Read the model definition and answer for the solid it produces. Units are mm, in the model's axes. Face numbers are marked on the shaded views. A direction names the side the tool comes from. Give positions to 0.01 mm unless a question says otherwise; leave off trailing zeros. Loops run counter-clockwise (first coordinate to the right, second up) from the corner with the lowest first, then second, coordinate; pieces in that order, holes last.
(1) Find section B-B, the plane x = 0. Write down the section's boundary in (y, z), then the cut area to 3 significant figures.
(2) Straight lines are drawn through the part: probe 1 along Y at (x, z) = (-12, -49.5); probe 2 along X at (y, z) = (-18, -48); probe 3 along X at (y, z) = (-12, -13.5). For each, find the intervals that lie inside material, in ascending order.
(3) Find section C-C, the plane x = -8.75. Write down the section's boundary in (y, z).
(4) Find section D-D, the plane y = -3.5. Write down the section's boundary in (x, z), then the cut area to 3 significant figures.
(5) Which of the six approach directions +Z, -Z, +X, -X, +Y, -Y give full straight-line access (tool end or side, diameter ignored) to the marked faces 1, 2, 3, 4 and 5?
(6) Determine the mould class of the marked faces 6, 7 and 8 for opening direction Z: pulls with the +Z half, pulls with the -Z half, needs draft (parallel to the pull), parting line crosses it, or undercut.
(7) Each of these flat-tipped pins is pushed along its axis until it touches: P1, Ø14.5, axis at x = 4, z = -47.5, coming from the +Y side; P2, Ø11, axis at x = -1.5, y = 14.5, coming from the +Z side; P3, Ø3, axis at x = -2.5, z = -17.5, coming from the -Y side; P4, Ø1, axis at x = -11.5, y = -13, coming from the +Z side. Where does it stop, or does it pass through?
(8) Find section A-A, the plane z = -35.5. Write down the section's boundary in (x, y).
```python
from build123d import *

# Parameters (mm, degrees)
SKETCH3_R           = 10
BOSS_EXTRUDE2_DEPTH = 12
BOSS_EXTRUDE3_DEPTH = 5
SKETCH5_R           = 15
BOSS_EXTRUDE4_DEPTH = 4
SKETCH6_W           = 30
SKETCH6_H           = 45
BOSS_EXTRUDE6_DEPTH = 10
BOSS_EXTRUDE7_START = 12.5
SKETCH7_R           = 8
BOSS_EXTRUDE7_DEPTH = 10
BOSS_EXTRUDE8_START = -22.5
SKETCH7_2_R         = 8
BOSS_EXTRUDE8_DEPTH = 10
CUT_EXTRUDE1_REACH  = 80.861


with BuildPart() as part:
    # Sketch3 → Boss-Extrude2 (new, symmetric)
    with BuildSketch(Plane(origin=(0, 0, 0), x_dir=(0, 0, -1), z_dir=(1, 0, 0))):
        Circle(SKETCH3_R)
    extrude(amount=BOSS_EXTRUDE2_DEPTH, both=True)

    # Sketch4 → Boss-Extrude3 (add, symmetric)
    with BuildSketch(Plane(origin=(0, 0, 0), x_dir=(0, 0, -1), z_dir=(1, 0, 0))):
        with BuildLine():
            Line((0, 14), (16, 14))
            Line((16, 14), (16, -14))
            Line((16, -14), (0, -14))
            ThreePointArc((0, -14), (-14, 0), (0, 14))
        make_face()
    extrude(amount=BOSS_EXTRUDE3_DEPTH, both=True)

    # Sketch5 → Boss-Extrude4 (add)
    with BuildSketch(Plane(origin=(0, 0, -16), x_dir=(-1, 0, 0), z_dir=(0, 0, -1))):
        Circle(SKETCH5_R)
    extrude(amount=BOSS_EXTRUDE4_DEPTH)

    # Sketch6 → Boss-Extrude6 (add)
    with BuildSketch(Plane(origin=(0, 0, -20), x_dir=(-1, 0, 0), z_dir=(0, 0, -1))):
        Rectangle(SKETCH6_W, SKETCH6_H)
    extrude(amount=BOSS_EXTRUDE6_DEPTH)

    # Sketch7 → Boss-Extrude7 (add)
    with BuildSketch(Plane(origin=(0, 0, 0), x_dir=(1, 0, 0), z_dir=(0, 1, 0)).offset(BOSS_EXTRUDE7_START)):
        with BuildLine():
            Line((-15, 30), (-15, 48))
            ThreePointArc((-15, 48), (0, 63), (15, 48))
            Line((15, 48), (15, 30))
            Line((15, 30), (-15, 30))
        make_face()
        with Locations(Location((0, 48, 0), (0, 0, 270))):
            Circle(SKETCH7_R, mode=Mode.SUBTRACT)
    extrude(amount=BOSS_EXTRUDE7_DEPTH)

    # Sketch7<2> → Boss-Extrude8 (add)
    with BuildSketch(Plane(origin=(0, 0, 0), x_dir=(1, 0, 0), z_dir=(0, 1, 0)).offset(BOSS_EXTRUDE8_START)):
        with BuildLine():
            Line((-15, 30), (-15, 48))
            ThreePointArc((-15, 48), (0, 63), (15, 48))
            Line((15, 48), (15, 30))
            Line((15, 30), (-15, 30))
        make_face()
        with Locations(Location((0, 48, 0), (0, 0, 270))):
            Circle(SKETCH7_2_R, mode=Mode.SUBTRACT)
    extrude(amount=BOSS_EXTRUDE8_DEPTH)

    # Cut-Extrude1: up to this face of the body (flat: up to its plane)
    cut_extrude1_end = Plane(part.part.faces().sort_by_distance((0, -22.5, -38.416854183))[0])
    # Sketch8 → Cut-Extrude1 (cut, up to the picked face)
    with BuildSketch(Plane(origin=(0, 22.5, 0), x_dir=(1, 0, 0), z_dir=(0, 1, 0)), mode=Mode.PRIVATE) as cut_extrude1_sk1:
        with BuildLine():
            Line((-9.909192751, 59.260901342), (-5.2849028, 54.005814049))
            ThreePointArc((-5.2849028, 54.005814049), (0, 56), (5.2849028, 54.005814049))
            Line((5.2849028, 54.005814049), (9.909192751, 59.260901342))
            ThreePointArc((9.909192751, 59.260901342), (0, 63), (-9.909192751, 59.260901342))
        make_face()
    cut_extrude1_tool1 = split(extrude(cut_extrude1_sk1.sketch, amount=-CUT_EXTRUDE1_REACH, mode=Mode.PRIVATE), bisect_by=cut_extrude1_end, keep=Keep.BOTH, mode=Mode.PRIVATE)
    add(cut_extrude1_tool1.solids().sort_by(Axis((0, 22.5, -58.852599), (0, -1, 0)))[0], mode=Mode.SUBTRACT)


solid = part.part
```
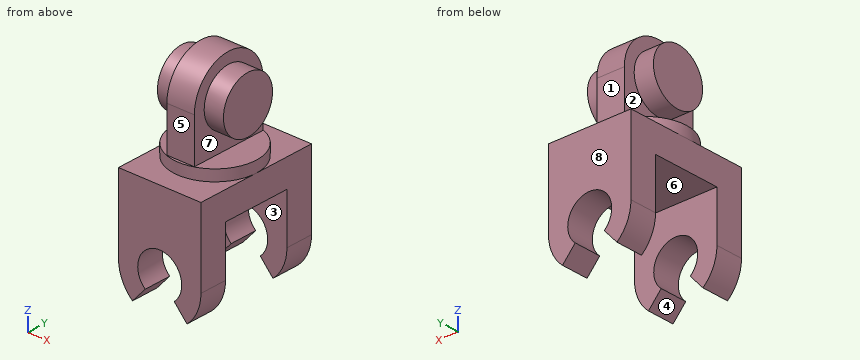
Entries:
1. outline: (-22.5, -40) - (-12.5, -40) - (-12.5, -30) - (12.5, -30) - (12.5, -40) - (22.5, -40) - (22.5, -20) - (15, -20) - (15, -16) - (14, -16) - (14, 0) arc R14 ccw to (-14, 0) - (-14, -16) - (-15, -16) - (-15, -20) - (-22.5, -20) - close
1. area: 1,530 mm2
2. probe 1: y = -22.5 to -12.5, 12.5 to 22.5
2. probe 2: x = -15 to -8, 8 to 15
2. probe 3: x = -5 to 5
3. outline: (-22.5, -57.94) - (-12.5, -57.94) - (-12.5, -30) - (12.5, -30) - (12.5, -57.94) - (22.5, -57.94) - (22.5, -20) - (12.18, -20) - (12.18, -16) - (-12.18, -16) - (-12.18, -20) - (-22.5, -20) - close; circle Ø20 at (0, 0)
4. outline: (-15, -30) - (15, -30) - (15, -20) - (14.59, -20) - (14.59, -16) - (5, -16) - (5, -9.37) - (12, -9.37) - (12, 9.37) - (5, 9.37) - (5, 13.56) - (-5, 13.56) - (-5, 9.37) - (-12, 9.37) - (-12, -9.37) - (-5, -9.37) - (-5, -16) - (-14.59, -16) - (-14.59, -20) - (-15, -20) - close
4. area: 975 mm2
5. face 1: +Z, +X, -X, +Y
5. face 2: -X
5. face 3: -Z, +X, -X
5. face 4: -Z, +Y, -Y
5. face 5: +Z, +X, -X, -Y
6. face 6: pulls with the -Z half
6. face 7: undercut
6. face 8: needs draft
7. P1: stops at y = 22.5
7. P2: stops at z = 10.72
7. P3: stops at y = -14.97
7. P4: stops at z = -20
8. outline: (-15, -22.5) - (15, -22.5) - (15, -12.5) - (-15, -12.5) - close; (-15, 12.5) - (15, 12.5) - (15, 22.5) - (-15, 22.5) - close
